from build123d import *

# Parameters (mm, degrees)
BOSS_EXTRUDE1_DEPTH  = 6
SOLENOID_PLACEMENT_W = 38
SOLENOID_PLACEMENT_H = 64
CUT_EXTRUDE1_DEPTH   = 103.528044944
CUT_EXTRUDE4_DEPTH   = 103.528044944
SKETCH5_R            = 12.5
CUT_EXTRUDE5_DEPTH   = 103.528044944
SKETCH6_R            = 2.4
CUT_EXTRUDE6_DEPTH   = 103.528044944
CUT_EXTRUDE3_DEPTH   = 103.528044944
FILLET1_R            = 2
CUT_EXTRUDE7_DEPTH   = 3
SKETCH10_R           = 5
CUT_EXTRUDE9_DEPTH   = 2
SKETCH11_W           = 69
SKETCH11_H           = 67
CUT_EXTRUDE10_DEPTH  = 99.059529102
SKETCH13_R           = 1.55
CUT_EXTRUDE11_DEPTH  = 4.2
SKETCH14_R           = 2.1
CUT_EXTRUDE12_DEPTH  = 9
SKETCH15_W           = 4
SKETCH15_H           = 10.882727098
CUT_EXTRUDE13_DEPTH  = 9
CIRPATTERN1_COUNT    = 3
CIRPATTERN1_ANGLE    = 120
CUT_EXTRUDE14_DEPTH  = 2.5
FILLET2_R            = 5


with BuildPart() as part:
    # Sketch1 → Boss-Extrude1 (new, symmetric)
    with BuildSketch(Plane(origin=(0, 0, 0), x_dir=(1, 0, 0), z_dir=(0, 1, 0))):
        with BuildLine():
            ThreePointArc((36.224522061, -62.223661106), (0, 72), (-36.224522061, -62.223661106))
            ThreePointArc((-36.224522061, -62.223661106), (-32.797800029, -62.818856853), (-29.811944095, -61.035223988))
            ThreePointArc((-29.811944095, -61.035223988), (0, -46.75), (29.811944095, -61.035223988))
            ThreePointArc((29.811944095, -61.035223988), (32.797800029, -62.818856853), (36.224522061, -62.223661106))
        make_face()
    extrude(amount=BOSS_EXTRUDE1_DEPTH, both=True)

    # solenoid placement → Cut-Extrude1 (cut, through all)
    with BuildSketch(Plane(origin=(0, 6, 0), x_dir=(1, 0, 0), z_dir=(0, 1, 0))):
        with Locations((0, -4)):
            Rectangle(SOLENOID_PLACEMENT_W, SOLENOID_PLACEMENT_H)
    extrude(amount=-CUT_EXTRUDE1_DEPTH, mode=Mode.SUBTRACT)

    # Sketch4 → Cut-Extrude4 (cut, through all)
    with BuildSketch(Plane(origin=(0, 6, 0), x_dir=(1, 0, 0), z_dir=(0, 1, 0))):
        with BuildLine():
            Line((-13, 28), (13, 28))
            Line((13, 28), (13, 43.2))
            ThreePointArc((13, 43.2), (12.414213562, 44.614213562), (11, 45.2))
            Line((11, 45.2), (-11, 45.2))
            ThreePointArc((-11, 45.2), (-12.414213562, 44.614213562), (-13, 43.2))
            Line((-13, 43.2), (-13, 28))
        make_face()
    extrude(amount=-CUT_EXTRUDE4_DEPTH, mode=Mode.SUBTRACT)

    # Sketch5 → Cut-Extrude5 (cut, through all)
    with BuildSketch(Plane(origin=(0, 6, 0), x_dir=(1, 0, 0), z_dir=(0, 1, 0))):
        with Locations(Location((27, 48, 0), (0, 0, 90))):
            Circle(SKETCH5_R)
        with Locations(Location((-27, 48, 0), (0, 0, 270))):
            Circle(SKETCH5_R)
    extrude(amount=-CUT_EXTRUDE5_DEPTH, mode=Mode.SUBTRACT)

    # Sketch6 → Cut-Extrude6 (cut, through all)
    with BuildSketch(Plane(origin=(0, 6, 0), x_dir=(1, 0, 0), z_dir=(0, 1, 0))):
        with Locations(Location((48, 40, 0), (0, 0, 90))):
            Circle(SKETCH6_R)
        with Locations(Location((-48, 40, 0), (0, 0, 270))):
            Circle(SKETCH6_R)
    extrude(amount=-CUT_EXTRUDE6_DEPTH, mode=Mode.SUBTRACT)

    # Sketch3 → Cut-Extrude3 (cut, through all)
    with BuildSketch(Plane(origin=(0, 6, 0), x_dir=(1, 0, 0), z_dir=(0, 1, 0))):
        Polygon((-72, -31.5), (-72, 27.5), (-59, 27.5), (-59, 31.5), (0, 31.5), (59, 31.5), (59, 27.5), (72, 27.5), (72, -31.5), (72, -101.646422462), (-72, -101.646422462), align=None)
    extrude(amount=-CUT_EXTRUDE3_DEPTH, mode=Mode.SUBTRACT)

    # Fillet1
    fillet1_edges = [part.edges().sort_by_distance(p)[0] for p in [
        (-66.541340534, 0, -27.5),
        (66.541340534, 0, -27.5),
        (-59, 0, -31.5),
        (59, 0, -31.5),
    ]]
    fillet(fillet1_edges, radius=FILLET1_R)

    # Sketch8 → Cut-Extrude7 (cut, symmetric)
    with BuildSketch(Plane(origin=(0, 0, 0), x_dir=(1, 0, 0), z_dir=(0, 1, 0))):
        with BuildLine():
            Line((5, 71.826179071), (5, 68.826179071))
            Line((5, 68.826179071), (-5, 68.826179071))
            Line((-5, 68.826179071), (-5, 71.826179071))
            ThreePointArc((-5, 71.826179071), (0, 72), (5, 71.826179071))
        make_face()
        with BuildLine():
            Line((64.703295733, 31.582962517), (62.105219521, 30.082962517))
            Line((62.105219521, 30.082962517), (57.105219521, 38.743216555))
            Line((57.105219521, 38.743216555), (59.703295733, 40.243216555))
            ThreePointArc((59.703295733, 40.243216555), (62.353829072, 36), (64.703295733, 31.582962517))
        make_face()
        with BuildLine():
            Line((-59.703295733, 40.243216555), (-57.105219521, 38.743216555))
            Line((-57.105219521, 38.743216555), (-62.105219521, 30.082962517))
            Line((-62.105219521, 30.082962517), (-64.703295733, 31.582962517))
            ThreePointArc((-64.703295733, 31.582962517), (-62.353829072, 36), (-59.703295733, 40.243216555))
        make_face()
    extrude(amount=CUT_EXTRUDE7_DEPTH, both=True, mode=Mode.SUBTRACT)

    # Sketch10 → Cut-Extrude9 (cut)
    with BuildSketch(Plane(origin=(0, 6, 0), x_dir=(1, 0, 0), z_dir=(0, 1, 0))):
        with Locations(Location((0, 55, 0), (0, 0, 270))):
            Circle(SKETCH10_R)
    extrude(amount=-CUT_EXTRUDE9_DEPTH, mode=Mode.SUBTRACT)

    # Sketch11 → Cut-Extrude10 (cut, through all)
    with BuildSketch(Plane(origin=(0, 6, 0), x_dir=(1, 0, 0), z_dir=(0, 1, 0))):
        Rectangle(SKETCH11_W, SKETCH11_H)
    extrude(amount=-CUT_EXTRUDE10_DEPTH, mode=Mode.SUBTRACT)

    # Sketch13 → Cut-Extrude11 (cut)
    with BuildSketch(Plane(origin=(-59.605219521, 0, -34.413089536), x_dir=(-0.5000000000000001, 0, 0.8660254037844386), z_dir=(-0.8660254037844386, 0, -0.5000000000000001))):
        Circle(SKETCH13_R)
    cut_extrude11 = extrude(amount=-CUT_EXTRUDE11_DEPTH, mode=Mode.SUBTRACT)

    # Sketch14 → Cut-Extrude12 (cut)
    with BuildSketch(Plane(origin=(-55.967912825, 0, -32.313089536), x_dir=(-0.5000000000000001, 0, 0.8660254037844386), z_dir=(-0.8660254037844386, 0, -0.5000000000000001))):
        Circle(SKETCH14_R)
    cut_extrude12 = extrude(amount=-CUT_EXTRUDE12_DEPTH, mode=Mode.SUBTRACT)

    # Sketch15 → Cut-Extrude13 (cut)
    with BuildSketch(Plane(origin=(-55.967912825, 0, -32.313089536), x_dir=(0.5000000000000001, 0, -0.8660254037844386), z_dir=(0.8660254037844386, 0, 0.5000000000000001))):
        with Locations((0, 5.441363549)):
            Rectangle(SKETCH15_W, SKETCH15_H)
    cut_extrude13 = extrude(amount=CUT_EXTRUDE13_DEPTH, mode=Mode.SUBTRACT)

    # CirPattern1: Cut-Extrude11, Cut-Extrude12, Cut-Extrude13 ×3 about axis
    cirpattern1_axis = Axis((0, 0, 0), (0, -1, 0))
    add([cut_extrude11.rotate(cirpattern1_axis, i * CIRPATTERN1_ANGLE / (CIRPATTERN1_COUNT - 1)) for i in range(1, CIRPATTERN1_COUNT)], mode=Mode.SUBTRACT)
    add([cut_extrude12.rotate(cirpattern1_axis, i * CIRPATTERN1_ANGLE / (CIRPATTERN1_COUNT - 1)) for i in range(1, CIRPATTERN1_COUNT)], mode=Mode.SUBTRACT)
    add([cut_extrude13.rotate(cirpattern1_axis, i * CIRPATTERN1_ANGLE / (CIRPATTERN1_COUNT - 1)) for i in range(1, CIRPATTERN1_COUNT)], mode=Mode.SUBTRACT)

    # Sketch16 → Cut-Extrude14 (cut)
    with BuildSketch(Plane(origin=(0, 6, 0), x_dir=(1, 0, 0), z_dir=(0, 1, 0))):
        with BuildLine():
            Line((-56.437350288, 31.5), (-60.621778265, 35))
            ThreePointArc((-60.621778265, 35), (0, 70), (60.621778265, 35))
            Line((60.621778265, 35), (56.477458213, 31.430531036))
            Line((56.477458213, 31.430531036), (53.977458213, 35.760658055))
            Line((53.977458213, 35.760658055), (55.69643641, 37.241199916))
            ThreePointArc((55.69643641, 37.241199916), (33.107279951, 58.248673927), (3.5, 66.908519637))
            Line((3.5, 66.908519637), (3.5, 55))
            Line((3.5, 55), (-3.5, 55))
            Line((-3.5, 55), (-3.5, 66.908519637))
            ThreePointArc((-3.5, 66.908519637), (-33.087061005, 58.260161295), (-55.670571638, 37.279853185))
            Line((-55.670571638, 37.279853185), (-53.937350288, 35.830127019))
            Line((-53.937350288, 35.830127019), (-56.437350288, 31.5))
        make_face()
    extrude(amount=-CUT_EXTRUDE14_DEPTH, mode=Mode.SUBTRACT)

    # Fillet2
    # the kernel refuses this fillet: 5 mm, written as the material it takes off along each edge
    with BuildSketch(Plane(origin=(55.69643641, 16.329932335, -37.241199916), x_dir=(-0.5812078308679164, 0, -0.8137551581021232), z_dir=(0, -1, 0))) as fillet2_piece_1:
        with BuildLine():
            CenterArc((3.97779484, -4.997622346), FILLET2_R, 88.232969076, 58.560507528)
            Line((-0.205714987, -2.259329899), (-0.289385184, -2.20456405))
            ThreePointArc((-0.289385184, -2.20456405), (-0.202445536, -1.120597326), (-0.099588042, 0.009067624))
            Line((-0.099588042, 0.009067624), (-0.003083562, 0.099952447))
            ThreePointArc((-0.003083562, 0.099952447), (2.065986467, 0.131860561), (4.135056496, 0.099952447))
            Line((4.135056496, 0.099952447), (4.131972934, 0))
        make_face()
    extrude(amount=12.829932335, mode=Mode.SUBTRACT)
    with BuildSketch(Plane(origin=(-3.5, 20.277950053, -66.908519637), x_dir=(-0.9955007283712978, 0, 0.09475389074975102), z_dir=(0, -1, 0))) as fillet2_piece_2:
        with BuildLine():
            CenterArc((5.498076289, -4.995456616), FILLET2_R, 87.557271181, 97.879883712)
            Line((0.520572647, -5.469226069), (0.421022574, -5.478701459))
            Line((0.421022574, -5.478701459), (-0.099550073, -0.009475389))
            Line((-0.099550073, -0.009475389), (-0.004262075, 0.099909132))
            ThreePointArc((-0.004262075, 0.099909132), (2.855590011, 0.16088135), (5.715442096, 0.099909132))
            Line((5.715442096, 0.099909132), (5.711180021, 0))
        make_face()
    extrude(amount=16.777950053, mode=Mode.SUBTRACT)
    with BuildSketch(Plane(origin=(3.5, 20.277950053, -66.908519637), x_dir=(0.9955007283712978, 0, 0.09475389074975099), z_dir=(0, -1, 0))) as fillet2_piece_3:
        with BuildLine():
            CenterArc((5.498076289, 4.995456616), FILLET2_R, 174.562845107, 97.879883712)
            Line((0.520572647, 5.469226069), (0.421022574, 5.478701459))
            Line((0.421022574, 5.478701459), (-0.099550073, 0.009475389))
            Line((-0.099550073, 0.009475389), (-0.004262075, -0.099909132))
            ThreePointArc((-0.004262075, -0.099909132), (2.855590011, -0.16088135), (5.715442096, -0.099909132))
            Line((5.715442096, -0.099909132), (5.711180021, 0))
        make_face()
    extrude(amount=16.777950053, mode=Mode.SUBTRACT)
    with BuildSketch(Plane(origin=(-55.670571638, 16.411618265, -37.279853185), x_dir=(0.581970971434149, 0, -0.8132095599585589), z_dir=(0, -1, 0))) as fillet2_piece_4:
        with BuildLine():
            CenterArc((4.009250019, 4.997584585), FILLET2_R, 213.290400287, 58.490608258)
            Line((-0.170246664, 2.253170717), (-0.253836598, 2.198282439))
            ThreePointArc((-0.253836598, 2.198282439), (-0.184839093, 1.119050965), (-0.099715761, -0.007534394))
            Line((-0.099715761, -0.007534394), (-0.003107946, -0.099951692))
            ThreePointArc((-0.003107946, -0.099951692), (2.082323653, -0.132366563), (4.167755252, -0.099951692))
            Line((4.167755252, -0.099951692), (4.164647306, 0))
        make_face()
    extrude(amount=12.911618265, mode=Mode.SUBTRACT)
    with BuildSketch(Plane(origin=(54.967912825, 15.964026198, -34.045140343), x_dir=(-0.8660254037844403, 0, 0.4999999999999973), z_dir=(0, -1, 0))) as fillet2_piece_5:
        with BuildLine():
            CenterArc((3.985610479, 5), FILLET2_R, 217.143845078, 52.856154922)
            Line((0, 1.980909225), (-0.07971221, 1.92052741))
            ThreePointArc((-0.07971221, 1.92052741), (-0.1, 0.990454613), (-0.1, 0))
            Line((-0.1, 0), (0, -0.1))
            Line((0, -0.1), (3.985610479, -0.1))
            Line((3.985610479, -0.1), (3.985610479, 0))
        make_face()
    extrude(amount=12.464026198, mode=Mode.SUBTRACT)
    with BuildSketch(Plane(origin=(-54.967912825, 3.5, -34.045140343), x_dir=(0.8660254037844386, 0, 0.5), z_dir=(0, 1, 0))) as fillet2_piece_6:
        with BuildLine():
            CenterArc((4.04512227, 5), FILLET2_R, 215.999272853, 54.000727147)
            Line((0, 2.061125075), (-0.080902445, 2.002347577))
            ThreePointArc((-0.080902445, 2.002347577), (-0.1, 1.030562538), (-0.1, 0))
            Line((-0.1, 0), (0, -0.1))
            Line((0, -0.1), (4.04512227, -0.1))
            Line((4.04512227, -0.1), (4.04512227, 0))
        make_face()
    extrude(amount=12.612805674, mode=Mode.SUBTRACT)


solid = part.part
Geometry: final body of the model. Coordinates: model frame, mm. A direction names the side the tool comes from. Give positions to 0.01 mm unless a question says otherwise; leave off trailing zeros. Write each loop counter-clockwise with the first axis right and the second up, starting at its lowest first coordinate (ties: lowest second). Pieces come first, ordered by that corner, then holes.
(1) First-contact query: P1, Ø2, axis at y = -1.5, z = -33, coming from the +X side; P2, Ø0.5, axis at x = -56.5, y = 4, coming from the +Z side; P3, Ø3.5, axis at x = -0.5, y = 1, coming from the +Z side. Flat tips, straight axial feed; report the tip coordinate or a pass-through.
(2) Ray query, line 1 (Y direction, x = 0, z = -65); line 2 (X direction, y = 2.5, z = -48); line 3 (X direction, y = -3.25, z = -38). Return the intervals inside material, ascending.
(3) Access query for faces 1 (the flat face through (0, 0, -45.2)), 2 (the flat face through (52.305, 2.687, -32.508)), 3 (the cylindrical face through (-19.286, 4.768, -64.164)). Directions: +Z, -Z, +X, -X, +Y, -Y. A direction counts if a zero-diameter tool reaches every point of the face in a straight line with its end or side. Return the directions, or none.
(4) Cut plane A-A, the plane x = 0. Return loops of the section in (y, z).
(5) Mould query, pull axis Y, two halves, no side actions, for faces 4 (the flat face through (0, 3, -70)), 5 (the cylindrical face through (57.073, 0.466, -34.658)), 6 (the flat face through (0, 3.5, -65)), 7 (the flat face through (-43, 0, -31.5)). Classes: released by +Y, released by -Y, zero draft, split by the parting line, or undercut.
(6) Cut plane C-C, the plane x = 41.5. Return loops of the section in (y, z), then the cut area to 3 significant figures.
(7) Cut plane B-B, the plane x = 16. Return loops of the section in (y, z).
Values follow:
1. P1: stops at x = 61
1. P2: stops at z = -31.5
1. P3: stops at z = -45.2
2. line 1: y = -6 to -1.55, 1.55 to 3.5
2. line 2: x = -53.67 to -39.5, -14.5 to 14.5, 39.5 to 53.67
2. line 3: x = -61.16 to -49.33, -46.67 to -34.5, -19.5 to -13, 13 to 19.5, 34.5 to 46.67, 49.33 to 61.16
3. face 1: +Z, +Y, -Y
3. face 2: +Z, +Y
3. face 3: +Y
4. outline: (-6, -72) - (-3, -72) - (-3, -68.83) - (-1.55, -68.83) - (-1.55, -64.63) - (-2.1, -64.63) - (-2.1, -55.63) - (3.5, -55.63) - (3.5, -55) - (4, -55) - (4, -50) - (6, -50) - (6, -45.2) - (-6, -45.2) - close; (1.55, -68.83) - (3, -68.83) - (3, -72) - (6, -72) - (6, -70) - (3.5, -70) - (3.5, -64.63) - (1.55, -64.63) - close
5. face 4: undercut
5. face 5: undercut
5. face 6: released by +Y
5. face 7: zero draft
6. outline: (-6, -58.84) - (6, -58.84) - (6, -56.37) - (3.5, -56.37) - (3.5, -52.6) - (6, -52.6) - (6, -31.5) - (-6, -31.5) - close
6. area: 319 mm2
7. outline: (-6, -70.2) - (6, -70.2) - (6, -68.15) - (3.5, -68.15) - (3.5, -65.06) - (6, -65.06) - (6, -53.94) - (-6, -53.94) - close; (-6, -42.06) - (6, -42.06) - (6, -33.5) - (-6, -33.5) - close
